Verification items for the finished model (mm, model axes). A direction names the side the tool comes from. Round coordinates to 2 decimals unless told otherwise and drop trailing zeros. Order: outer loops, then holes, each group sorted by start corner. A loop starts at its lowest first (then second) coordinate and runs counter-clockwise, first axis right, second up. Notation, with made-up numbers: (52, 80) -> (101, 80) arc R12 cw to (101, 101) -> close; hole circle Ø1 at (68.5, 3). An arc over 180 degrees is marked (long way). Put each result on its own line as item: value.
from build123d import *

# Parameters (mm, degrees)
F0_R     = 30
F0_R_2   = 25
F1_DEPTH = 1120
F0_R_3   = 82.5
F0_R_4   = 9
F2_DEPTH = 15
F3_R     = 82.5
F3_R_2   = 9
F3_R_3   = 30
F4_DEPTH = 15
F5_R     = 50
F5_R_2   = 25
F6_DEPTH = 3


with BuildPart() as f1:
    # F0 (on Front) → F1 (new body)
    with BuildSketch(Plane.XZ):
        Circle(F0_R)
        Circle(F0_R_2, mode=Mode.SUBTRACT)
    extrude(amount=F1_DEPTH)

    # F0 (on Front) → F2 (join)
    with BuildSketch(Plane.XZ):
        Circle(F0_R_3)
        with Locations((0, -62.5)):
            Circle(F0_R_4, mode=Mode.SUBTRACT)
        with Locations((-62.5, 0)):
            Circle(F0_R_4, mode=Mode.SUBTRACT)
        Circle(F0_R, mode=Mode.SUBTRACT)
        with Locations((62.5, 0)):
            Circle(F0_R_4, mode=Mode.SUBTRACT)
        with Locations((0, 62.5)):
            Circle(F0_R_4, mode=Mode.SUBTRACT)
    extrude(amount=F2_DEPTH)

    # F3 (on face) → F4 (join)
    with BuildSketch(Plane.XZ.offset(1120)):
        Circle(F3_R)
        with Locations((0, -62.5)):
            Circle(F3_R_2, mode=Mode.SUBTRACT)
        with Locations((-62.5, 0)):
            Circle(F3_R_2, mode=Mode.SUBTRACT)
        Circle(F3_R_3, mode=Mode.SUBTRACT)
        with Locations((62.5, 0)):
            Circle(F3_R_2, mode=Mode.SUBTRACT)
        with Locations((0, 62.5)):
            Circle(F3_R_2, mode=Mode.SUBTRACT)
    extrude(amount=-F4_DEPTH)

    # F5 (on face) → F6 (join)
    with BuildSketch(Plane.XZ.offset(1120)):
        Circle(F5_R)
        Circle(F5_R_2, mode=Mode.SUBTRACT)
    extrude(amount=F6_DEPTH)


solid = f1.part
Item 1: Section check A-A on y = -1010.5. Record the boundary of the cut face in (x, z).
Check sheet entries:
outline: circle Ø60 at (0, 0); hole circle Ø50 at (0, 0)
Item 2: Material ranges on L1, parallel to Z at x = 0, y = -1111.5; L2, parallel to Y at x = 44, z = -56; L3, parallel to X at y = -847, z = 3, recorded low to high. Write a range as [from, to].
Check sheet entries:
L1: z = [-82.5, -71.5], [-53.5, -25], [25, 53.5], [71.5, 82.5]
L2: y = [-1120, -1105], [-15, 0]
L3: x = [-29.85, -24.82], [24.82, 29.85]
Item 3: Release check for a two-part mould opening along X. For faces 4 (the cylindrical face through (-1.951, -1112.605, 53.714)), 5 (the flat face through (-22.9, -1123, -10.4)), 6 (the cylindrical face through (-17.88, -1112.6, -80.54)) record: +X half, -X half, draft (parallel to the pull), parting line (faces both ways), or undercut.
Check sheet entries:
face 4: undercut
face 5: draft
face 6: parting line
Item 4: Tool access check on faces 1 (the cylindrical face through (-29.97, -552.37, 1.32)), 2 (the cylindrical face through (71.084, -1112.605, 2.703)), 3 (the flat face through (36, -1120, -36)). Record the directions out of +Z, -Z, +X, -X, +Y, -Y that give a thin tool (end or side, any length) a straight path to the whole face; none if there is none.
Check sheet entries:
face 1: none
face 2: +Y, -Y
face 3: -Y
Item 5: Gauge pin test, flat ends, axial feed: pin 1 Ø3 at (x, y) = (-7, -352.5) entering from +Z; pin 2 Ø11 at (x, z) = (0, 62.5) entering from -Y; pin 3 Ø1 at (x, z) = (44.5, -48.5) entering from -Y; pin 4 Ø12 at (y, z) = (-774.5, 19) entering from -X. Record the tip position at first contact, or that the pin passes through.
Check sheet entries:
pin 1: stops at z = 29.49
pin 2: passes through
pin 3: stops at y = -1120
pin 4: stops at x = -27.04
